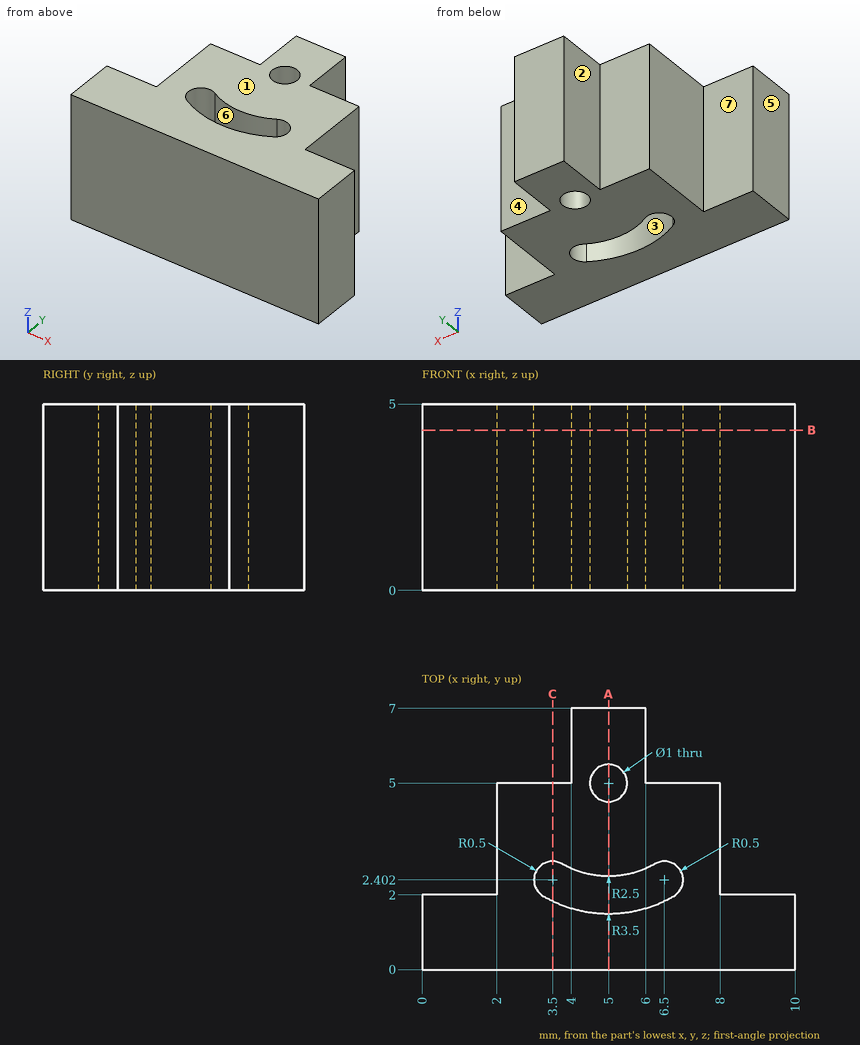
Here's the drawing with two shaded views (mm, measured from the low corner). I have some questions. A direction names the side the tool comes from. Round coordinates to 2 decimals unless told otherwise and drop trailing zeros. Order: outer loops, then holes, each group sorted by start corner. A loop starts at its lowest first (then second) coordinate and runs counter-clockwise, first axis right, second up. Notation, with made-up numbers: (71, 28) -> (124, 28) arc R14 cw to (124, 41) -> close; hole circle Ø3 at (25.5, 5). An arc over 180 degrees is marked (long way). Write each question's results on one line, items separated by ' | '. Start each with the question number.
Item 1: If we section it at A-A, the plane x = 5: Write out the boundary of the cut face in (y, z), then the cut area to 3 significant figures.
Item 2: Thinking about a two-plate mould opening in Y: for the marked faces 5, 6 and 7, which applies, +Y half, -Y half, draft (parallel to the pull), parting line (faces both ways), or undercut?
Item 3: Which directions (+Z, -Z, +X, -X, +Y, -Y) give clear straight access to the entire face, cutting with the end or side of a thin tool? Please do the marked faces 1, 2, 3 and 4.
Item 4: Please list where these lines run through material, in increasing order: L1, parallel to Y at x = 5, z = 4.05; L2, parallel to X at y = 6.5, z = 2.4; L3, parallel to Y at x = 2.5, z = 2.75.
Item 5: If we section it at C-C, the plane x = 3.5: Write out the boundary of the cut face in (y, z).
Item 6: Will these pins go through, and if not, where does the flat tip stop? pin 1 (1 mm diameter, centred on x = 6.5, z = 1, fed in from -Y); pin 2 (0.9 mm diameter, centred on y = 3.5, z = 2, fed in from +X); pin 3 (1 mm diameter, centred on x = 7, z = 2.5, fed in from +Y); pin 4 (0.6 mm diameter, centred on x = 9, z = 1.5, fed in from +Y).
Item 7: If we section it at B-B, the plane z = 4.3: Write out the boundary of the cut face in (x, y) (3 decimals), then the cut area to 3 significant figures.
Results:
1) outline: (0, 0) -> (1.5, 0) -> (1.5, 5) -> (0, 5) -> close; (2.5, 0) -> (4.5, 0) -> (4.5, 5) -> (2.5, 5) -> close; (5.5, 0) -> (7, 0) -> (7, 5) -> (5.5, 5) -> close | area: 25.0 mm2
2) face 5: draft | face 6: undercut | face 7: +Y half
3) face 1: +Z, +X, -X, +Y, -Y | face 2: +Z, -Z, -X, +Y | face 3: +Z, -Z | face 4: +Z, -Z, +X, +Y
4) L1: y = 0 to 1.5, 2.5 to 4.5, 5.5 to 7 | L2: x = 4 to 6 | L3: y = 0 to 5
5) outline: (0, 0) -> (1.84, 0) -> (1.84, 5) -> (0, 5) -> close; (2.9, 0) -> (5, 0) -> (5, 5) -> (2.9, 5) -> close
6) pin 1: stops at y = 0 | pin 2: stops at x = 8 | pin 3: stops at y = 5 | pin 4: stops at y = 2
7) outline: (0, 0) -> (10, 0) -> (10, 2) -> (8, 2) -> (8, 5) -> (6, 5) -> (6, 7) -> (4, 7) -> (4, 5) -> (2, 5) -> (2, 2) -> (0, 2) -> close; hole (3.25, 1.969) arc R3.5 ccw to (6.75, 1.969) arc R0.5 ccw to (6.25, 2.835) arc R2.5 cw to (3.75, 2.835) arc R0.5 ccw to start; hole circle Ø1 at (5, 5) | area: 37.3 mm2
